```python
from build123d import *

# Parameters (mm, degrees)
CYLINDER030_R     = 4.55
CYLINDER030_DEPTH = 10
CYLINDER029_R     = 1.4
CYLINDER029_DEPTH = 10
ARRAY002_COUNT    = 3
CYLINDER031_R     = 4.1
CYLINDER031_DEPTH = 10
BOX002_W          = 10
BOX002_H          = 5
BOX002_DEPTH      = 1.5875
FILLET001_R       = 2
ARRAY003_COUNT    = 3
CYLINDER032_R     = 7
CYLINDER032_DEPTH = 1.59


with BuildPart() as mountplatelip001:
    # Cylinder030 → Cylinder030 (new body)
    with BuildSketch(Plane.XY.offset(0.6)):
        Circle(CYLINDER030_R)
    extrude(amount=CYLINDER030_DEPTH)


with BuildPart() as array002:
    # Cylinder029 → Cylinder029 (new body)
    with BuildSketch(Plane(origin=(8, 0, 0), x_dir=(1, 0, 0), z_dir=(0, 0, 1))):
        Circle(CYLINDER029_R)
    extrude(amount=CYLINDER029_DEPTH)

    # Array002: Array002 ×3 about axis
    array002_axis = Axis((0, 0, 0), (0, 0, 1))


with BuildPart() as array002_1:
    add(array002.part)
    for i in range(1, ARRAY002_COUNT):
        add(array002.part.rotate(array002_axis, i * 360 / ARRAY002_COUNT))


with BuildPart() as fusion006:
    # Cylinder031 → Cylinder031 (new body)
    with BuildSketch(Plane.XY):
        Circle(CYLINDER031_R)
    extrude(amount=CYLINDER031_DEPTH)

    # Fusion006: union MountPlateLip001, Array002
    add(mountplatelip001.part)
    add(array002_1.part)


with BuildPart() as array003:
    # Box002 → Box002 (new body)
    with BuildSketch(Plane(origin=(0.5, -2.5, 0), x_dir=(1, 0, 0), z_dir=(0, 0, 1))):
        with Locations((5, 2.5)):
            Rectangle(BOX002_W, BOX002_H)
    extrude(amount=BOX002_DEPTH)

    # Fillet001
    fillet001_edges = [array003.edges().sort_by_distance(p)[0] for p in [
        (10.5, -2.5, 0.79375),
        (10.5, 2.5, 0.79375),
    ]]
    fillet(fillet001_edges, radius=FILLET001_R)

    # Array003: Array003 ×3 about axis
    array003_axis = Axis((0, 0, 0), (0, 0, 1))


with BuildPart() as array003_1:
    add(array003.part)
    for i in range(1, ARRAY003_COUNT):
        add(array003.part.rotate(array003_axis, i * 360 / ARRAY003_COUNT))


with BuildPart() as cut009:
    # Cylinder032 → Cylinder032 (new body)
    with BuildSketch(Plane.XY):
        Circle(CYLINDER032_R)
    extrude(amount=CYLINDER032_DEPTH)

    # Fusion007: union Array003
    add(array003_1.part)

    # Cut009: cut Fusion006
    add(fusion006.part, mode=Mode.SUBTRACT)


solid = cut009.part
```
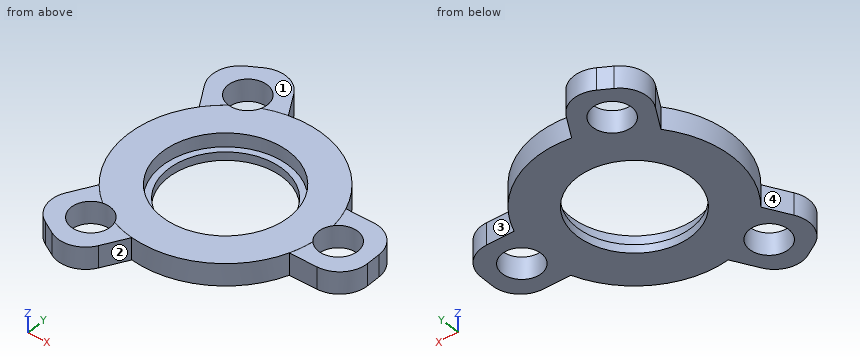
Design review of the part built by this model. Coordinates are the model's own, in mm. Face numbers are marked on the shaded views. Coordinates: 2 decimals unless noted, no trailing zeros. Loops run counter-clockwise (first coordinate to the right, second up) from the corner with the lowest first, then second, coordinate; pieces in that order, holes last. Notation, with made-up numbers: (53, -16.75) -> (106, -16.75) arc R18 ccw to (106, -0.75) -> close; hole circle Ø5 at (10.5, 67). An arc over 180 degrees is marked (long way). Answer as a JSON object with one key per item and string values.
Q1. Take a section at D-D on x = 8. Give the boundary of the cut face in (y, z).
Answer block:
{"outline": "(-2.5, 0) -> (-1.4, 0) -> (-1.4, 1.59) -> (-2.5, 1.59) -> close; (1.4, 0) -> (2.5, 0) -> (2.5, 1.59) -> (1.4, 1.59) -> close"}
Q2. The part is to be moulded in two halves that separate along Y. For the marked faces 1, 2, 3 and 4, say which applies: +Y half, -Y half, draft (parallel to the pull), parting line (faces both ways), or undercut.
Answer block:
{"face 1": "draft", "face 2": "-Y half", "face 3": "+Y half", "face 4": "undercut"}
Q3. Clearance check with flat-ended pins moving along their axes: pin 1 Ø0.8 at (x, z) = (7.5, 1) entering from -Y; pin 2 Ø4.5 at (x, y) = (2, 0.5) entering from +Z. State where each tip first meets the part, or that it passes through.
Answer block:
{"pin 1": "stops at y = -2.5", "pin 2": "stops at z = 0.6"}
Q4. Take a section at C-C on z = 0.35. Give the boundary of the cut face in (x, y).
Answer block:
{"outline": "(-6.42, -6.11) arc R2 ccw to (-5.68, -8.84) -> (-4.82, -9.34) arc R2 ccw to (-2.08, -8.61) -> (-1.1, -6.91) arc R7 ccw to (6.54, -2.5) -> (8.5, -2.5) arc R2 ccw to (10.5, -0.5) -> (10.5, 0.5) arc R2 ccw to (8.5, 2.5) -> (6.54, 2.5) arc R7 ccw to (-1.1, 6.91) -> (-2.08, 8.61) arc R2 ccw to (-4.82, 9.34) -> (-5.68, 8.84) arc R2 ccw to (-6.42, 6.11) -> (-5.43, 4.41) arc R7 ccw to (-5.43, -4.41) -> close; hole circle Ø2.8 at (-4, -6.93); hole circle Ø2.8 at (-4, 6.93); hole circle Ø8.2 at (0, 0); hole circle Ø2.8 at (8, 0)"}
Q5. Take a section at B-B on y = 0. Give the boundary of the cut face in (x, z), plus the area to 3 significant figures.
Answer block:
{"outline": "(-7, 0) -> (-4.1, 0) -> (-4.1, 0.6) -> (-4.55, 0.6) -> (-4.55, 1.59) -> (-7, 1.59) -> close; (4.1, 0) -> (6.6, 0) -> (6.6, 1.59) -> (4.55, 1.59) -> (4.55, 0.6) -> (4.1, 0.6) -> close; (9.4, 0) -> (10.5, 0) -> (10.5, 1.59) -> (9.4, 1.59) -> close", "area": "9.44 mm^2"}
Q6. To check wall thickness, follow L1, parallel to X at y = 0, z = 0.2; L2, parallel to Y at x = 8, z = 0.5; L3, parallel to X at y = 0.25, z = 0.9. State the ranges of each line that lie inside material, in increasing order.
Answer block:
{"L1": "x = -7 to -4.1, 4.1 to 6.6, 9.4 to 10.5", "L2": "y = -2.5 to -1.4, 1.4 to 2.5", "L3": "x = -7 to -4.54, 4.54 to 6.62, 9.38 to 10.5"}
Q7. Take a section at A-A on x = 0. Give the boundary of the cut face in (y, z), plus the area to 3 significant figures.
Answer block:
{"outline": "(-7, 0) -> (-4.1, 0) -> (-4.1, 0.6) -> (-4.55, 0.6) -> (-4.55, 1.59) -> (-7, 1.59) -> close; (4.1, 0) -> (7, 0) -> (7, 1.59) -> (4.55, 1.59) -> (4.55, 0.6) -> (4.1, 0.6) -> close", "area": "8.33 mm^2"}
